```python
from build123d import *

# Parameters (mm, degrees)
SKETCH1_R                       = 25.4
BOSS_EXTRUDE1_DEPTH             = 33
CUT_EXTRUDE1_DEPTH              = 34
SKETCH3_R                       = 25.4
SKETCH3_R_2                     = 23
CUT_EXTRUDE2_DEPTH              = 15
M3X0_5_TAPPED_HOLE1_D           = 2.5
M3X0_5_TAPPED_HOLE1_DEPTH       = 25
M3X0_5_TAPPED_HOLE1_CSINK_D     = 3.05
M3X0_5_TAPPED_HOLE1_CSINK_ANGLE = 90
M3X0_5_TAPPED_HOLE1_TIP         = 0.751075774
SKETCH6_W                       = 55.513598287
SKETCH6_H                       = 26.495126455
CUT_EXTRUDE3_DEPTH              = 15


with BuildPart() as part:
    # Sketch1 → Boss-Extrude1 (new body)
    with BuildSketch(Plane.XY):
        Circle(SKETCH1_R)
    extrude(amount=BOSS_EXTRUDE1_DEPTH)

    # Sketch2 → Cut-Extrude1 (cut, through all)
    with BuildSketch(Plane.XY.offset(33)):
        with BuildLine():
            Line((-21.5, 0), (-10.6, 0))
            Line((-10.6, 0), (-10.6, -20))
            Line((-10.6, -20), (10.6, -20))
            Line((10.6, -20), (10.6, 0))
            Line((10.6, 0), (21.5, 0))
            ThreePointArc((21.5, 0), (0, 21.5), (-21.5, 0))
        make_face()
    extrude(amount=-CUT_EXTRUDE1_DEPTH, mode=Mode.SUBTRACT)

    # Sketch3 → Cut-Extrude2 (cut)
    with BuildSketch(Plane(origin=(0, 0, 0), x_dir=(-1, 0, 0), z_dir=(0, 0, -1))):
        Circle(SKETCH3_R)
        Circle(SKETCH3_R_2, mode=Mode.SUBTRACT)
    extrude(amount=-CUT_EXTRUDE2_DEPTH, mode=Mode.SUBTRACT)

    # M3x0.5 Tapped Hole1
    with Locations(Plane(origin=(-23.868192568, 8.68731164, 0), x_dir=(0, 0, -1), z_dir=(-0.939692621, 0.342020143, 0))):
        with Locations((-27, 10), (-15.5, 10), (-6, 10)):
            CounterSinkHole(M3X0_5_TAPPED_HOLE1_D / 2, M3X0_5_TAPPED_HOLE1_CSINK_D / 2, depth=M3X0_5_TAPPED_HOLE1_DEPTH, counter_sink_angle=M3X0_5_TAPPED_HOLE1_CSINK_ANGLE)
            with Locations((0, 0, -(M3X0_5_TAPPED_HOLE1_DEPTH + M3X0_5_TAPPED_HOLE1_TIP / 2))):  # 118° drill point
                Cone(0, M3X0_5_TAPPED_HOLE1_D / 2, M3X0_5_TAPPED_HOLE1_TIP, mode=Mode.SUBTRACT)

    # Sketch6 → Cut-Extrude3 (cut)
    with BuildSketch(Plane(origin=(0, 0, 0), x_dir=(-1, 0, 0), z_dir=(0, 0, -1))):
        with Locations((1.479202462, 13.247563228)):
            Rectangle(SKETCH6_W, SKETCH6_H)
    extrude(amount=-CUT_EXTRUDE3_DEPTH, mode=Mode.SUBTRACT)


solid = part.part
```
Could you check a few things on this model? Use its own coordinates, in mm. A direction names the side the tool comes from. Coordinates: 2 decimals unless noted, no trailing zeros. Loops run counter-clockwise (first coordinate to the right, second up) from the corner with the lowest first, then second, coordinate; pieces in that order, holes last.
1) Thinking about a two-plate mould opening in Z: for faces 1 (the face through (12, -8, 0)), 2 (the face through (0.473, 21.495, 24.126)), 3 (the face through (-17.078, -5.745, 5.837)), which applies, released by +Z, released by -Z, zero draft, split by the parting line, or undercut?
Reported:
face 1: released by -Z
face 2: zero draft
face 3: undercut
2) Imagine slicing it at B-B (z = 9.5). List the corners of the cut face in (x, y) for me.
Reported:
outline: (-23, 0) arc R23 ccw to (23, 0) - (10.6, 0) - (10.6, -20) - (-10.6, -20) - (-10.6, 0) - close
3) Will these pins go through, and if not, where does the flat tip stop? pin 1 Ø1.5 at (x, z) = (16, 17.5) entering from +Y; pin 2 Ø3 at (x, z) = (-9, 23) entering from -Y; pin 3 Ø3 at (y, z) = (17, 19.5) entering from +X.
Reported:
pin 1: stops at y = 20.31
pin 2: stops at y = -24.27
pin 3: stops at x = 20.12
4) Imagine slicing it at C-C (x = -18.5). State how many separate pieces and enclosed holes the cut face has, and give its area (3 significant figures).
Reported:
separate pieces: 2
enclosed holes: 3
area: 619 mm2
5) Imagine slicing it at A-A (x = 0). List the corners of the cut face in (y, z) for me, and give its area (3 significant figures).
Reported:
outline: (-25.4, 15) - (-23, 15) - (-23, 0) - (-20, 0) - (-20, 33) - (-25.4, 33) - close; (21.5, 15) - (25.4, 15) - (25.4, 33) - (21.5, 33) - close
area: 212 mm2
6) Imagine slicing it at D-D (x = 14). List the corners of the cut face in (y, z) for me.
Reported:
outline: (-21.19, 15) - (-18.25, 15) - (-18.25, 0) - (0, 0) - (0, 33) - (-21.19, 33) - close; (16.32, 15) - (21.19, 15) - (21.19, 33) - (16.32, 33) - close
7) Which directions (+Z, -Z, +X, -X, +Y, -Y) give clear straight access to the entire face, cutting with the end or side of a thin tool? Please do faces 4 (the face through (0.506, -22.994, 7.395)), 5 (the face through (0, -20, 17)), 6 (the face through (11, -5, 33)).
Reported:
face 4: -Z, -Y
face 5: +Z, -Z
face 6: +Z, +X, -X, +Y, -Y
8) Please list where these lines run through material, in increasing order: line 1 along Z through (x, y) = (-22.5, 4); line 2 along X through (y, z) = (-1.5, 20); line 3 along X through (y, z) = (17.5, 23).
Reported:
line 1: z = 15 to 33
line 2: x = -25.36 to -10.6, 10.6 to 25.36
line 3: x = -18.41 to -12.49, 12.49 to 18.41
